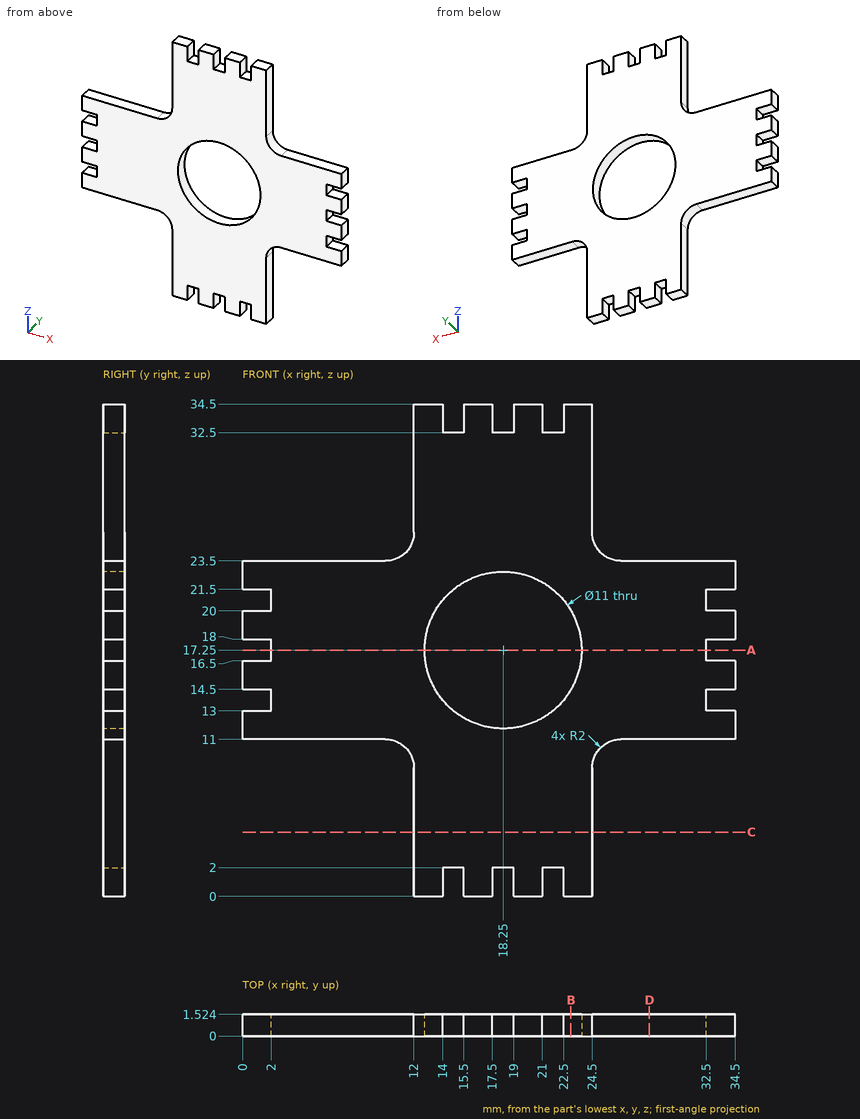
Part print with two shaded views. Sizes in mm from the minimum x, y, z corner. Coordinates: 2 decimals unless noted, no trailing zeros. Write each loop counter-clockwise with the first axis right and the second up, starting at its lowest first coordinate (ties: lowest second). Pieces come first, ordered by that corner, then holes. Notation, with made-up numbers: M 6.25,6.5 L 46.25,6.5 A18 cw 46.25,25.5 Z; hole C 19.5,-31.5 d5. An arc over 180 degrees is marked long. Return JSON: item names as keys, results as strings.
Item 1: Slice it at A-A, the plane z = 17.25. Write the cut outline in (x, y), and give its area (3 significant figures).
Findings below:
{"outline": "M 2,0 L 12.75,0 L 12.75,1.52 L 2,1.52 Z; M 23.75,0 L 32.5,0 L 32.5,1.52 L 23.75,1.52 Z", "area": "29.7 mm2"}
Item 2: Probe line 1 (Z direction, x = 18.25, y = 0.45); line 2 (X direction, y = 0.95, z = 17.5); line 3 (Z direction, x = 27, y = 1.05). List the from-to ranges inside material, lowest first. Write a range as from..to.
Findings below:
{"line 1": "z = 2..11.75, 22.75..32.5", "line 2": "x = 2..12.76, 23.74..32.5", "line 3": "z = 11..23.5"}
Item 3: Slice it at C-C, the plane z = 4.5. Write the cut outline in (x, y), and give its area (4 significant figures).
Findings below:
{"outline": "M 12,0 L 24.5,0 L 24.5,1.52 L 12,1.52 Z", "area": "19.05 mm2"}
Item 4: Slice it at B-B, the plane x = 23. Write the cut outline in (y, z), and give its area (3 significant figures).
Findings below:
{"outline": "M 0,0 L 1.52,0 L 1.52,14.48 L 0,14.48 Z; M 0,20.02 L 1.52,20.02 L 1.52,34.5 L 0,34.5 Z", "area": "44.1 mm2"}
Item 5: Drop flat-ended pins along their axis: pin 1 Ø0.5 at (y, z) = (0.5, 30.5) entering from +X; pin 2 Ø0.5 at (y, z) = (0.5, 33) entering from -X; pin 3 Ø0.8 at (y, z) = (1, 21) entering from -X. Give the stop position or say it passes through.
Findings below:
{"pin 1": "stops at x = 24.5", "pin 2": "stops at x = 12", "pin 3": "stops at x = 2"}
Item 6: Slice it at D-D, the plane x = 28.5. Write the cut outline in (y, z), and give its area (4 significant figures).
Findings below:
{"outline": "M 0,11 L 1.52,11 L 1.52,23.5 L 0,23.5 Z", "area": "19.05 mm2"}
